Could you check a few things on this model? Use its own coordinates, in mm. A direction names the side the tool comes from. Round coordinates to 2 decimals unless told otherwise and drop trailing zeros. Loops run counter-clockwise (first coordinate to the right, second up) from the corner with the lowest first, then second, coordinate; pieces in that order, holes last. Notation, with made-up numbers: (63, -36.5) -> (109, -36.5) arc R26 ccw to (109, 1.5) -> close; hole circle Ø8 at (51.25, 18). An arc over 180 degrees is marked (long way). One line per item, written item: value.
from build123d import *

# Parameters (mm, degrees)
BOSS_EXTRUDE1_DEPTH = 120
SKETCH2_W           = 8
SKETCH2_H           = 8
BOSS_EXTRUDE2_DEPTH = 48
CUT_EXTRUDE1_REACH  = 135.147
SKETCH3_R           = 3
SKETCH4_W           = 48
SKETCH4_H           = 24
BOSS_EXTRUDE3_DEPTH = 3
SKETCH5_W           = 4.321078357
SKETCH5_H           = 3
BOSS_EXTRUDE4_DEPTH = 5
SKETCH6_R           = 0.75
CUT_EXTRUDE2_DEPTH  = 129.842888822
BOSS_EXTRUDE5_DEPTH = 20


with BuildPart() as part:
    # Sketch1 → Boss-Extrude1 (new body)
    with BuildSketch(Plane(origin=(0, 0, 0), x_dir=(0, 0, -1), z_dir=(1, 0, 0))):
        with BuildLine():
            Line((21, 0), (24, 0))
            Line((24, 0), (24, -24))
            Line((24, -24), (-24, -24))
            Line((-24, -24), (-24, 0))
            Line((-24, 0), (-21, 0))
            ThreePointArc((-21, 0), (0, -21), (21, 0))
        make_face()
    extrude(amount=BOSS_EXTRUDE1_DEPTH)

    # Sketch2 → Boss-Extrude2 (add)
    with BuildSketch(Plane.XY.offset(24)):
        with Locations((4, -28)):
            Rectangle(SKETCH2_W, SKETCH2_H)
    extrude(amount=-BOSS_EXTRUDE2_DEPTH)

    # Sketch3 → Cut-Extrude1 (cut, up to next)
    with BuildSketch(Plane.XY.offset(24), mode=Mode.PRIVATE) as cut_extrude1_sk1:
        with Locations((4, -27.835840809)):
            Circle(SKETCH3_R)
    cut_extrude1_tool1 = extrude(cut_extrude1_sk1.sketch, amount=-CUT_EXTRUDE1_REACH, mode=Mode.PRIVATE) & part.part
    add(cut_extrude1_tool1.solids().sort_by_distance((4, -27.835841, 24))[0], mode=Mode.SUBTRACT)

    # Sketch4 → Boss-Extrude3 (add)
    with BuildSketch(Plane(origin=(120, 0, 0), x_dir=(0, 0, -1), z_dir=(1, 0, 0))):
        with Locations((0, -12)):
            Rectangle(SKETCH4_W, SKETCH4_H)
    extrude(amount=-BOSS_EXTRUDE3_DEPTH)

    # Sketch5 → Boss-Extrude4 (add)
    with BuildSketch(Plane.XZ.offset(24)):
        with Locations((17.531080317, -11.8)):
            Rectangle(SKETCH5_W, SKETCH5_H)
    extrude(amount=BOSS_EXTRUDE4_DEPTH)

    # Sketch6 → Cut-Extrude2 (cut, through all)
    with BuildSketch(Plane.XY.offset(-10.3)):
        with Locations((17.531080317, -26.5)):
            Circle(SKETCH6_R)
    extrude(amount=-CUT_EXTRUDE2_DEPTH, mode=Mode.SUBTRACT)

    # Sketch7 → Boss-Extrude5 (add)
    with BuildSketch(Plane(origin=(0, 0, 0), x_dir=(1, 0, 0), z_dir=(0, 1, 0))):
        Polygon((120, 24), (0, 24), (0, 21), (117, 21), (117, -21), (0, -21), (0, -24), (120, -24), align=None)
    extrude(amount=BOSS_EXTRUDE5_DEPTH)


solid = part.part
(1) Thinking about a two-plate mould opening in X: for faces 5 (the face through (58, -21, 0)), 6 (the face through (1.62, -29.66, 0.34)), 7 (the face through (15.371, -26, -12)), 8 (the face through (120, -2, 0)), which applies, released by +X, released by -X, zero draft, split by the parting line, or undercut?
Recorded:
face 5: zero draft
face 6: undercut
face 7: undercut
face 8: released by +X
(2) If we section it at A-A, the plane x = 4: Please give me the cut outline in (y, z), then the cut area to 3 significant figures.
Recorded:
outline: (-32, -24) -> (-30.84, -24) -> (-30.84, 24) -> (-32, 24) -> close; (-24.84, -24) -> (20, -24) -> (20, -21) -> (0, -21) arc R21 cw to (0, 21) -> (20, 21) -> (20, 24) -> (-24.84, 24) -> close
area: 675 mm²
(3) If we section it at B-B, the plane x = 94: Please give me the cut outline in (y, z), then the cut area to 3 significant figures.
Recorded:
outline: (-24, -24) -> (20, -24) -> (20, -21) -> (0, -21) arc R21 cw to (0, 21) -> (20, 21) -> (20, 24) -> (-24, 24) -> close
area: 579 mm²
(4) I'm going to push flat-ended pins straight in: pin 1 Ø2.5 at (x, y) = (17.53, -26.5) entering from -Z; pin 2 Ø5 at (y, z) = (-6, -5) entering from -X; pin 3 Ø3.5 at (x, z) = (17.5, -11.5) entering from -Y. Where does each tip first touch, or does it pass through?
Recorded:
pin 1: z = -13.3
pin 2: x = 117
pin 3: y = -29
(5) If I drill on L1, parallel to Z at x = 114, y = 8.5; L2, parallel to X at y = -26, z = -12; L3, parallel to Y at x = 99.5, z = 0.5, over which ranges is the centre line in solid material (lowest first)?
Recorded:
L1: -24 to -21, 21 to 24
L2: 0 to 1.63, 6.37 to 8, 15.37 to 16.97, 18.09 to 19.69
L3: -24 to -20.99
(6) If we section it at C-C, the plane z = 19: Please give me the cut outline in (x, y).
Recorded:
outline: (0, -32) -> (8, -32) -> (8, -24) -> (120, -24) -> (120, 20) -> (117, 20) -> (117, -8.94) -> (0, -8.94) -> close; hole circle Ø6 at (4, -27.84)
(7) For faces 1 (the face through (16.5, -26.5, -13.3)), 2 (the face through (16.5, -26.5, -10.3)), 3 (the face through (18, -29, -12)), 4 (the face through (117, -1, 0)), which set-ups out of +Z, -Z, +X, -X, +Y, -Y let a thin tool reach every point of the face, with its end or its side?
Recorded:
face 1: -Z, +X, -Y
face 2: +Z, +X, -Y
face 3: +Z, -Z, +X, -Y
face 4: -X, +Y
(8) If we section it at D-D, the plane y = -19: Please give me the cut outline in (x, z).
Recorded:
outline: (0, -24) -> (120, -24) -> (120, 24) -> (0, 24) -> (0, 8.94) -> (117, 8.94) -> (117, -8.94) -> (0, -8.94) -> close
